```python
from build123d import *

# Parameters (mm, degrees)
SKETCH1_R           = 2.4892
BOSS_EXTRUDE1_DEPTH = 3.175


with BuildPart() as part:
    # Sketch1 → Boss-Extrude1 (new body)
    with BuildSketch(Plane.XY.offset(3.175)):
        with BuildLine():
            Line((-6.519754617, 6.842706409), (9.448686805, 0.228361402))
            ThreePointArc((9.448686805, 0.228361402), (10.011466136, 0.057644159), (10.596737102, 0))
            Line((10.596737102, 0), (82.657359313, 0))
            ThreePointArc((82.657359313, 0), (83.80540961, 0.228361402), (84.778679656, 0.878679656))
            Line((84.778679656, 0.878679656), (88.021320344, 4.121320344))
            ThreePointArc((88.021320344, 4.121320344), (88.671638598, 5.09459039), (88.9, 6.242640687))
            Line((88.9, 6.242640687), (88.9, 19.157359313))
            ThreePointArc((88.9, 19.157359313), (88.671638598, 20.30540961), (88.021320344, 21.278679656))
            Line((88.021320344, 21.278679656), (84.778679656, 24.521320344))
            ThreePointArc((84.778679656, 24.521320344), (83.80540961, 25.171638598), (82.657359313, 25.4))
            Line((82.657359313, 25.4), (52.701598941, 25.4))
            ThreePointArc((52.701598941, 25.4), (49.775244111, 25.688220794), (46.961347456, 26.541807012))
            Line((46.961347456, 26.541807012), (-14.438795516, 51.974578963))
            ThreePointArc((-14.438795516, 51.974578963), (-17.032097526, 53.360727766), (-19.305145749, 55.226170233))
            Line((-19.305145749, 55.226170233), (-40.487067043, 76.408091527))
            ThreePointArc((-40.487067043, 76.408091527), (-41.460337089, 77.058409781), (-42.608387387, 77.286771184))
            Line((-42.608387387, 77.286771184), (-47.194173824, 77.286771184))
            ThreePointArc((-47.194173824, 77.286771184), (-48.342224121, 77.058409781), (-49.315494168, 76.408091527))
            Line((-49.315494168, 76.408091527), (-58.447579285, 67.27600641))
            ThreePointArc((-58.447579285, 67.27600641), (-59.097897539, 66.302736363), (-59.326258942, 65.154686066))
            Line((-59.326258942, 65.154686066), (-59.326258942, 60.568899629))
            ThreePointArc((-59.326258942, 60.568899629), (-59.097897539, 59.420849332), (-58.447579285, 58.447579285))
            Line((-58.447579285, 58.447579285), (-7.493024663, 7.493024663))
            ThreePointArc((-7.493024663, 7.493024663), (-7.038415019, 7.11993617), (-6.519754617, 6.842706409))
        make_face()
        with Locations((0, 17.960512242)):
            Circle(SKETCH1_R, mode=Mode.SUBTRACT)
        with Locations((12.7, 12.7)):
            Circle(SKETCH1_R, mode=Mode.SUBTRACT)
        with Locations((63.5, 12.7)):
            Circle(SKETCH1_R, mode=Mode.SUBTRACT)
        with Locations((38.1, 12.7)):
            Circle(SKETCH1_R, mode=Mode.SUBTRACT)
        with Locations((-17.960512242, 35.921024484)):
            Circle(SKETCH1_R, mode=Mode.SUBTRACT)
        with Locations((-35.921024484, 53.881536726)):
            Circle(SKETCH1_R, mode=Mode.SUBTRACT)
        with Locations((76.2, 12.7)):
            Circle(SKETCH1_R, mode=Mode.SUBTRACT)
        with Locations((50.8, 12.7)):
            Circle(SKETCH1_R, mode=Mode.SUBTRACT)
        with Locations((25.4, 12.7)):
            Circle(SKETCH1_R, mode=Mode.SUBTRACT)
        with Locations((-8.980256121, 26.940768363)):
            Circle(SKETCH1_R, mode=Mode.SUBTRACT)
        with Locations((-26.940768363, 44.901280605)):
            Circle(SKETCH1_R, mode=Mode.SUBTRACT)
        with Locations((-44.901280605, 62.861792847)):
            Circle(SKETCH1_R, mode=Mode.SUBTRACT)
    extrude(amount=-BOSS_EXTRUDE1_DEPTH)


solid = part.part
```
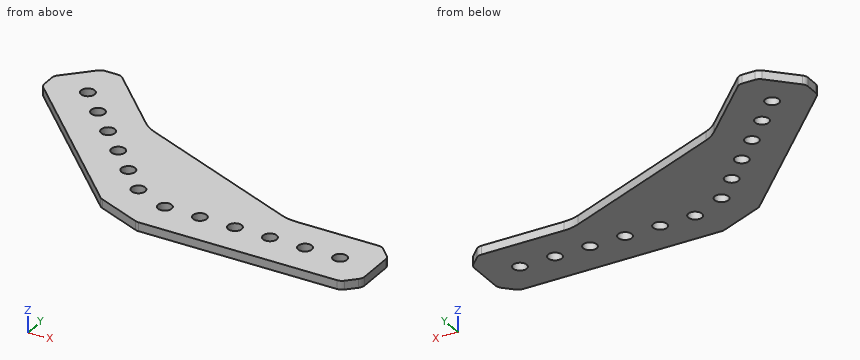
Verification items for the finished model (mm, model axes). Give positions to 0.01 mm unless a question says otherwise; leave off trailing zeros. Loops run counter-clockwise (first coordinate to the right, second up) from the corner with the lowest first, then second, coordinate; pieces in that order, holes last.
1. Thickness scan on line 1 (X direction, y = 46, z = 0.55); line 2 (X direction, y = 27.5, z = 1.5); line 3 (Y direction, x = 47, z = 2.9). Record the ranges inside material, lowest first.
2. Section check B-B, the plane x = 76.2. Enter the section's corners in (y, z) (3 decimals).
3. Go/stop test with flat-tipped pins: pin 1 Ø5.5 at (x, y) = (-17.96, 35.92) entering from +Z (3 decimals); pin 2 Ø1 at (x, z) = (70.5, 1) entering from +Y; pin 3 Ø3 at (x, y) = (25.4, 12.7) entering from +Z; pin 4 Ø1.5 at (y, z) = (60.5, 0.5) entering from +X. Record where each tip stops, or that it passes through.
4. Section check C-C, the plane z = 1.3. Count the separate pieces of the cut face and the enclosed holes in it, then the cut area to 3 significant figures.
5. Section check D-D, the plane x = 0. Enter the section's corners in (y, z) (3 decimals).
6. Section check A-A, the plane y = 12.7. Enter the section's corners in (x, z) (3 decimals), then the cut area to 3 significant figures.
Geometry says:
1. line 1: x = -46 to -29.17, -24.71 to -0.01
1. line 2: x = -27.5 to -11.41, -6.55 to 44.65
1. line 3: y = 0 to 26.53
2. outline: (0, 0) - (10.211, 0) - (10.211, 3.175) - (0, 3.175) - close; (15.189, 0) - (25.4, 0) - (25.4, 3.175) - (15.189, 3.175) - close
3. pin 1: stops at z = 3.175
3. pin 2: stops at y = 25.4
3. pin 3: passes through
3. pin 4: stops at x = -23.83
4. separate pieces: 1
4. enclosed holes: 12
4. area: 4,470 mm2
5. outline: (4.142, 0) - (15.471, 0) - (15.471, 3.175) - (4.142, 3.175) - close; (20.45, 0) - (45.994, 0) - (45.994, 3.175) - (20.45, 3.175) - close
6. outline: (-12.7, 0) - (10.211, 0) - (10.211, 3.175) - (-12.7, 3.175) - close; (15.189, 0) - (22.911, 0) - (22.911, 3.175) - (15.189, 3.175) - close; (27.889, 0) - (35.611, 0) - (35.611, 3.175) - (27.889, 3.175) - close; (40.589, 0) - (48.311, 0) - (48.311, 3.175) - (40.589, 3.175) - close; (53.289, 0) - (61.011, 0) - (61.011, 3.175) - (53.289, 3.175) - close; (65.989, 0) - (73.711, 0) - (73.711, 3.175) - (65.989, 3.175) - close; (78.689, 0) - (88.9, 0) - (88.9, 3.175) - (78.689, 3.175) - close
6. area: 228 mm2
